Read the model definition and answer for the solid it produces. Units are mm, in the model's axes. Give positions to 0.01 mm unless a question says otherwise; leave off trailing zeros. Write each loop counter-clockwise with the first axis right and the second up, starting at its lowest first coordinate (ties: lowest second). Pieces come first, ordered by that corner, then holes. Notation, with made-up numbers: (34.25, 72) -> (75.25, 72) arc R15 ccw to (75.25, 97) -> close; hole circle Ø10 at (76, 89.5). An arc over 180 degrees is marked (long way). Answer as CSV lines item,"result". Start each with the question number.
1. The part is cut by section B-B, the plane x = 20. Determine the outline of the cut face in (y, z).
2. The part is cut by section A-A, the plane z = 220.25. Determine the outline of the cut face in (x, y), and give its area (3 significant figures).
3. Given pin 1 (1 mm diameter, centred on y = -9, z = 175, fed in from -X); pin 2 (5.5 mm diameter, centred on x = 69.85, z = 6.35, fed in from -Y); pin 3 (5 mm diameter, centred on y = -2.5, z = 148.5, fed in from -X); pin 4 (4 mm diameter, centred on y = -3.5, z = 75.5, fed in from -X), each flat-ended and moving along its own axis, determine where each tip first touches the part or whether it passes through.
4. The part is cut by section C-C, the plane x = 38.1. Determine the outline of the cut face in (y, z) (3 decimals), and give its area (3 significant figures).
5. Find the intervals of material crossed by line 1 (Z direction, x = 80.01, y = -4.75) (3 decimals); line 2 (Y direction, x = 84.25, z = 233); line 3 (X direction, y = -5.25, z = 60.5), in increasing order.
from build123d import *

# Parameters (mm, degrees)
F1_DEPTH = 12.7
F2_R     = 2.54
F4_D     = 6.8
F4_DEPTH = 16.45
F4_TIP   = 2.0429261047
F6_D     = 5.1054
F6_DEPTH = 12.7
F6_TIP   = 1.5338169022
F8_D     = 6.7564


with BuildPart() as f1:
    # F0 (on Front) → F1 (new body)
    with BuildSketch(Plane.XZ):
        Polygon((0, 25.4), (0, 0), (88.9, 0), (88.9, 12.7), (88.9, 226.6), (88.9, 239.3), (88.9, 252), (74.1228589826, 252), align=None)
        Polygon((76.2, 217.5006349499), (76.2, 12.7), (12.7, 12.7), (12.7, 23.3756349499), align=None, mode=Mode.SUBTRACT)
        Polygon((76.4077141017, 258.985), (74.1228589826, 252), (88.9, 252), (88.9, 258.985), align=None)
    extrude(amount=F1_DEPTH)

    # F2
    f2_edges = [f1.edges().sort_by_distance(p)[0] for p in [
        (0, -6.35, 25.4),
        (76.2, -6.35, 12.7),
        (12.7, -6.35, 12.7),
        (12.7, -6.35, 23.375635),
        (76.2, -6.35, 217.500635),
        (76.407714, -6.35, 258.985),
    ]]
    fillet(f2_edges, radius=F2_R)

    # F4
    with Locations(Plane.YZ.offset(88.9)):
        with Locations((-6.35, 233), (-6.35, 19)):
            Hole(F4_D / 2, depth=F4_DEPTH)
            with Locations((0, 0, -(F4_DEPTH + F4_TIP / 2))):  # 118° drill point
                Cone(0, F4_D / 2, F4_TIP, mode=Mode.SUBTRACT)

    # F6
    with Locations(Plane(origin=(0, 0, 0), x_dir=(-1, 0, 0), z_dir=(0, 1, 0))):
        with Locations((-80.01, 245.65), (-80.01, 220.25)):
            Hole(F6_D / 2, depth=F6_DEPTH)
            with Locations((0, 0, -(F6_DEPTH + F6_TIP / 2))):  # 118° drill point
                Cone(0, F6_D / 2, F6_TIP, mode=Mode.SUBTRACT)

    # F8 (through all)
    with Locations(Plane.XZ.offset(12.7)):
        with Locations((6.35, 6.35), (38.1, 6.35), (69.85, 6.35)):
            Hole(F8_D / 2)


solid = f1.part
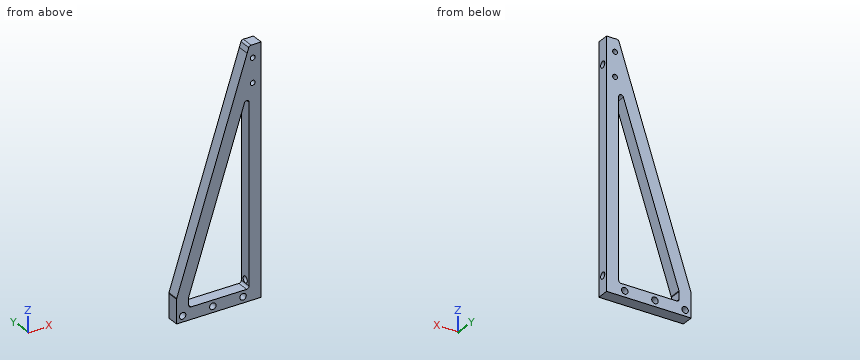
Results found:
1,outline,"(-12.7, 0) -> (0, 0) -> (0, 12.7) -> (-12.7, 12.7) -> close; (-12.7, 45.69) -> (0, 45.69) -> (0, 86.54) -> (-12.7, 86.54) -> close"
2,outline,"(63.74, -12.7) -> (77.46, -12.7) -> (77.46, 0) -> (63.74, 0) -> close; (82.56, -12.7) -> (88.9, -12.7) -> (88.9, 0) -> (82.56, 0) -> close"
2,area,"255 mm²"
3,pin 1,"stops at x = 48.77"
3,pin 2,"passes through"
3,pin 3,"stops at x = 39.45"
3,pin 4,"stops at x = 15.73"
4,outline,"(-12.7, 0) -> (0, 0) -> (0, 2.972) -> (-12.7, 2.972) -> close; (-12.7, 9.728) -> (0, 9.728) -> (0, 12.7) -> (-12.7, 12.7) -> close; (-12.7, 101.026) -> (0, 101.026) -> (0, 141.875) -> (-12.7, 141.875) -> close"
4,area,"594 mm²"
5,line 1,"z = 0 to 16, 22 to 217.697, 222.803 to 230, 236 to 243.097, 248.203 to 258.985"
5,line 2,"y = -12.7 to -9.75, -2.95 to 0"
5,line 3,"x = 11.48 to 24.84, 76.2 to 88.9"
